Could you check a few things on this model? Use its own coordinates, in mm. Face numbers are marked on the shaded views. A direction names the side the tool comes from. Give positions to 0.01 mm unless a question says otherwise; leave off trailing zeros. Write each loop counter-clockwise with the first axis right and the second up, starting at its lowest first coordinate (ties: lowest second). Pieces come first, ordered by that corner, then holes. Notation, with made-up numbers: M 17.5,-29.5 L 56.5,-29.5 A33 cw 56.5,4.5 Z; hole C -16.5,37.25 d8. An arc over 180 degrees is marked long. Use one line per item in the form item = value.
from build123d import *

# Parameters (mm, degrees)
F1_W     = 15
F1_H     = 10
F2_DEPTH = 1
F3_R     = 2.75
F4_DEPTH = 2
F6_DEPTH = 4
F7_R     = 2
F8_R     = 0.5


with BuildPart() as f2:
    # F1 (on Top) → F2 (new body)
    with BuildSketch(Plane.XY):
        Rectangle(F1_W, F1_H)
    extrude(amount=F2_DEPTH)

    # F3 (on Front) → F4 (join, symmetric)
    with BuildSketch(Plane.XZ):
        with Locations((0, 3)):
            Circle(F3_R)
    extrude(amount=F4_DEPTH, both=True)

    # F5 (on face) → F6 (cut, through all)
    with BuildSketch(Plane.XZ.offset(2)):
        with BuildLine():
            ThreePointArc((-1.4, 4.05), (-0.5533985905, 1.3398042284), (1.75, 3))
            ThreePointArc((1.75, 3), (1.6601957716, 3.5533985905), (1.4, 4.05))
            Line((1.4, 4.05), (1.4, 3.103264831))
            Line((1.4, 3.103264831), (-1.4, 3.103264831))
            Line((-1.4, 3.103264831), (-1.4, 4.05))
        make_face()
        with BuildLine():
            Line((1.4, 3.103264831), (1.4, 4.05))
            ThreePointArc((1.4, 4.05), (0, 4.75), (-1.4, 4.05))
            Line((-1.4, 4.05), (-1.4, 3.103264831))
            Line((-1.4, 3.103264831), (1.4, 3.103264831))
        make_face()
        with BuildLine():
            ThreePointArc((-1.4, 4.05), (0, 4.75), (1.4, 4.05))
            Line((1.4, 4.05), (1.4, 5.3669600757))
            ThreePointArc((1.4, 5.3669600757), (0, 5.75), (-1.4, 5.3669600757))
            Line((-1.4, 5.3669600757), (-1.4, 4.05))
        make_face()
    extrude(amount=-F6_DEPTH, mode=Mode.SUBTRACT)

    # F7
    f7_edges = [f2.edges().sort_by_distance(p)[0] for p in [
        (-1.887459, 0, 1),
        (1.887459, 0, 1),
    ]]
    fillet(f7_edges, radius=F7_R)

    # F8
    f8_edges = [f2.edges().sort_by_distance(p)[0] for p in [
        (-1.4, 0, 5.36696),
        (1.4, 0, 5.36696),
    ]]
    fillet(f8_edges, radius=F8_R)


solid = f2.part
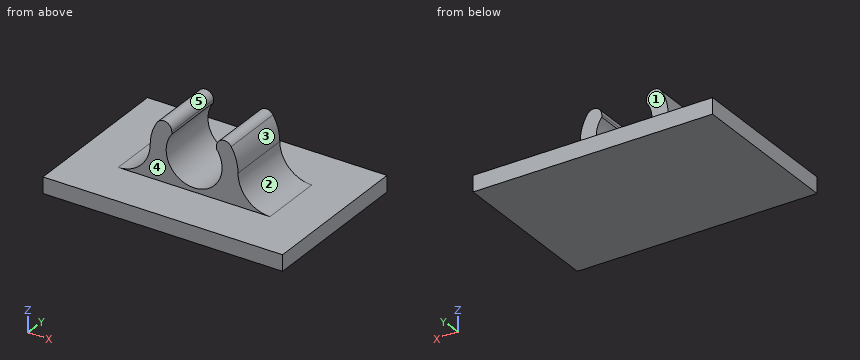
1) I want a section at A-A, the plane z = 3.9. Please give me the cut outline in (x, y), plus the area to 3 significant figures.
Checked values:
outline = M -2.6,-2 L -1.5,-2 L -1.5,2 L -2.6,2 Z; M 1.5,-2 L 2.6,-2 L 2.6,2 L 1.5,2 Z
area = 8.78 mm2
2) I want a section at C-C, the plane y = 1.75. Please give me the cut outline in (x, z).
Checked values:
outline = M -7.5,0 L 7.5,0 L 7.5,1 L 4.75,1 A2 cw 2.75,3 A2.75 ccw 2.32,4.47 A0.5 ccw 1.4,4.21 L 1.4,4.05 A1.75 cw long -1.4,4.05 L -1.4,4.21 A0.5 ccw -2.32,4.47 A2.75 ccw -2.75,3 A2 cw -4.75,1 L -7.5,1 Z
3) If I drill on L1, parallel to Z at x = 0, y = -2.25; L2, parallel to Z at x = 0, y = -0.4; L3, parallel to X at y = -1.75, z = 2.7, over which ranges is the centre line in solid material (lowest first)?
Checked values:
L1 = 0 to 1
L2 = 0 to 1.25
L3 = -2.77 to -1.72, 1.72 to 2.77
4) I want a section at B-B, the plane x = 0. Please give me the cut outline in (y, z), plus the area to 3 significant figures.
Checked values:
outline = M -5,0 L 5,0 L 5,1 L 2,1 L 2,1.25 L -2,1.25 L -2,1 L -5,1 Z
area = 11.0 mm2
5) For the marked faces 1 and 2, which set-ups out of +Z, -Z, +X, -X, +Y, -Y let a thin tool reach every point of the face, with its end or its side?
Checked values:
face_1 = +Z, +X, -X, +Y
face_2 = +Z, +X, +Y, -Y
6) I want a section at D-D, the plane z = 2.85. Please give me the cut outline in (x, y), plus the area to 3 significant figures.
Checked values:
outline = M -2.76,-2 L -1.74,-2 L -1.74,2 L -2.76,2 Z; M 1.74,-2 L 2.76,-2 L 2.76,2 L 1.74,2 Z
area = 8.10 mm2
7) Thinking about a two-plate mould opening in X: for the marked faces 3, 4 and 5, which applies, released by +X, released by -X, zero draft, split by the parting line, or undercut?
Checked values:
face_3 = released by +X
face_4 = zero draft
face_5 = undercut
8) For pin 1 Ø3 at (x, y) = (-1.5, -1.5) entering from +Z; pin 2 Ø1 at (x, y) = (-3, -1) entering from +Z; pin 3 Ø1.1 at (x, z) = (2, 2.5) entering from -Y, each with a flat end and sliding along its axis, tell me the tip position at first contact or that it passes through.
Checked values:
pin_1 = 4.71
pin_2 = 4.15
pin_3 = -2
